from build123d import *

# Parameters (mm, degrees)
F0_R     = 19.05
F1_DEPTH = 3.175
F2_R     = 14.986
F3_DEPTH = 5.08
F4_R     = 15.875
F5_DEPTH = 5.08
F6_SIZE2 = 5.07999
F6_SIZE  = 2.53999
F7_DEPTH = 10.16


# Not quite as in the source:
# - a fillet or chamfer is up to 0.001 mm smaller than in the source, because OpenCascade refuses the exact size


with BuildPart() as f1:
    # F0 (on Top) → F1 (new body)
    with BuildSketch(Plane.XY):
        Circle(F0_R)
    extrude(amount=F1_DEPTH)

    # F2 (on face) → F3 (join)
    with BuildSketch(Plane.XY.offset(3.175)):
        Circle(F2_R)
    extrude(amount=F3_DEPTH)

    # F4 (on face) → F5 (join)
    with BuildSketch(Plane.XY.offset(8.255)):
        Circle(F4_R)
    extrude(amount=F5_DEPTH)

    # F6 (size 2.54 and 5.08 in the source; OpenCascade refuses exactly that, so slightly less here)
    f6_edges = [f1.edges().sort_by_distance(p)[0] for p in [
        (-15.875, 0, 13.335),
    ]]
    f6_side = f1.faces().sort_by_distance((0, 0, 13.335))[0]
    chamfer(f6_edges, length=F6_SIZE, length2=F6_SIZE2, reference=f6_side)

    # F7 (cut): a face of the model
    f7_faces = [f1.faces().sort_by_distance(p)[0] for p in [
        (0, 0, 13.335),
    ]]
    extrude(f7_faces, amount=-F7_DEPTH, mode=Mode.SUBTRACT)


solid = f1.part
Part model, mm, in its own coordinate system. A direction names the side the tool comes from. Coordinates: 2 decimals unless noted, no trailing zeros. Loops run counter-clockwise (first coordinate to the right, second up) from the corner with the lowest first, then second, coordinate; pieces in that order, holes last. Notation, with made-up numbers: (-39, 48) -> (-22, 48) arc R28 cw to (-22, 71) -> close; hole circle Ø10 at (81, 78.5). An arc over 180 degrees is marked (long way). Use a Markdown table: item, result. Add a question column.
Item 1: Pull direction Z, two halves, no side cores. Call faces 1 (the flat face through (14, -6, 8.255)), 2 (the conical face through (12.87, 4.05, 13.02)), 3 (the cylindrical face through (7.169, 11.244, 8.326)), 4 (the flat face through (0, 0, 0)): +Z half, -Z half, draft (parallel to the pull), parting line (faces both ways), or undercut.
Item 2: Flat gauge pins, fed straight in: P1, Ø1.5, axis at y = 3, z = 9.5, coming from the +X side; P2, Ø1, axis at x = 3, y = 8, coming from the +Z side (3 decimals). Where does each tip first touch, or does it go through?
Item 3: Band-saw the part on C-C on z = 6. Write the cut outline in (x, y) (3 decimals).
Item 4: Probe probe 1 along Y at (x, z) = (0, 6) (3 decimals); probe 2 along Z at (x, y) = (0, -2) (3 decimals); probe 3 along Y at (x, z) = (-4.5, 4.5). List the from-to ranges inside material, lowest first.
Item 5: Which spindle directions (+Z, -Z, +X, -X, +Y, -Y) get a long thin tool onto all of the face, cutting with end or side? Do faces 5 (the cylindrical face through (-15.12, -11.59, 1.57)), 6 (the flat face through (0, 0, 3.175)), 7 (the flat face through (8, -13, 3.175)). Say none if no direction does.
Geometry says:
| question | item | result |
|---|---|---|
| 1 | face 1 | undercut |
| 1 | face 2 | +Z half |
| 1 | face 3 | draft |
| 1 | face 4 | -Z half |
| 2 | P1 | x = 15.36 |
| 2 | P2 | z = 3.175 |
| 3 | outline | circle Ø29.972 at (0, 0); hole circle Ø26.67 at (0, 0) |
| 4 | probe 1 | -14.986 to -13.335, 13.335 to 14.986 |
| 4 | probe 2 | 0 to 3.175 |
| 4 | probe 3 | -14.29 to -12.55, 12.55 to 14.29 |
| 5 | face 5 | +Z, -Z |
| 5 | face 6 | +Z |
| 5 | face 7 | none |
